The drawing under review shows one solid part. Ordinate dimensions are in mm from its lowest x, y, z. A direction names the side the tool comes from. Round coordinates to 2 decimals unless told otherwise and drop trailing zeros. Write each loop counter-clockwise with the first axis right and the second up, starting at its lowest first coordinate (ties: lowest second). Pieces come first, ordered by that corner, then holes. Notation, with made-up numbers: (66, 57.5) -> (89, 57.5) arc R11 cw to (89, 71.5) -> close; hole circle Ø7 at (-13, 52.25). An arc over 180 degrees is marked (long way). Write item = value, one per line. Start each with the question number.
Item 1: Add section B-B, the plane z = 9.5. State the section outline as (x, y) points, then the cut area to 3 significant figures.
Item 2: Add section C-C, the plane y = 21. State the section outline as (x, z) points.
Item 3: Add section A-A, the plane y = 50. State the section outline as (x, z) points, then the cut area to 3 significant figures.
Item 4: Mouldability with a two-part tool opening along Z and no side actions: class the marked faces 3, 4, 5 and 6 as released by +Z, released by -Z, zero draft, split by the parting line, or undercut.
Item 5: Machinability: for the marked faces 1 and 2, which of the approach directions +Z, -Z, +X, -X, +Y, -Y give a long, thin tool a straight path to every point of the face, cutting with its end or side? Answer none if there is none.
Item 6: To check wall thickness, follow L1, parallel to Z at x = 4.25, y = 21.5; L2, parallel to Z at x = 0.85, y = 50. State the ranges of each line that lie inside material, in increasing order.
Item 7: Add section D-D, the plane x = 9.5. State the section outline as (y, z) points.
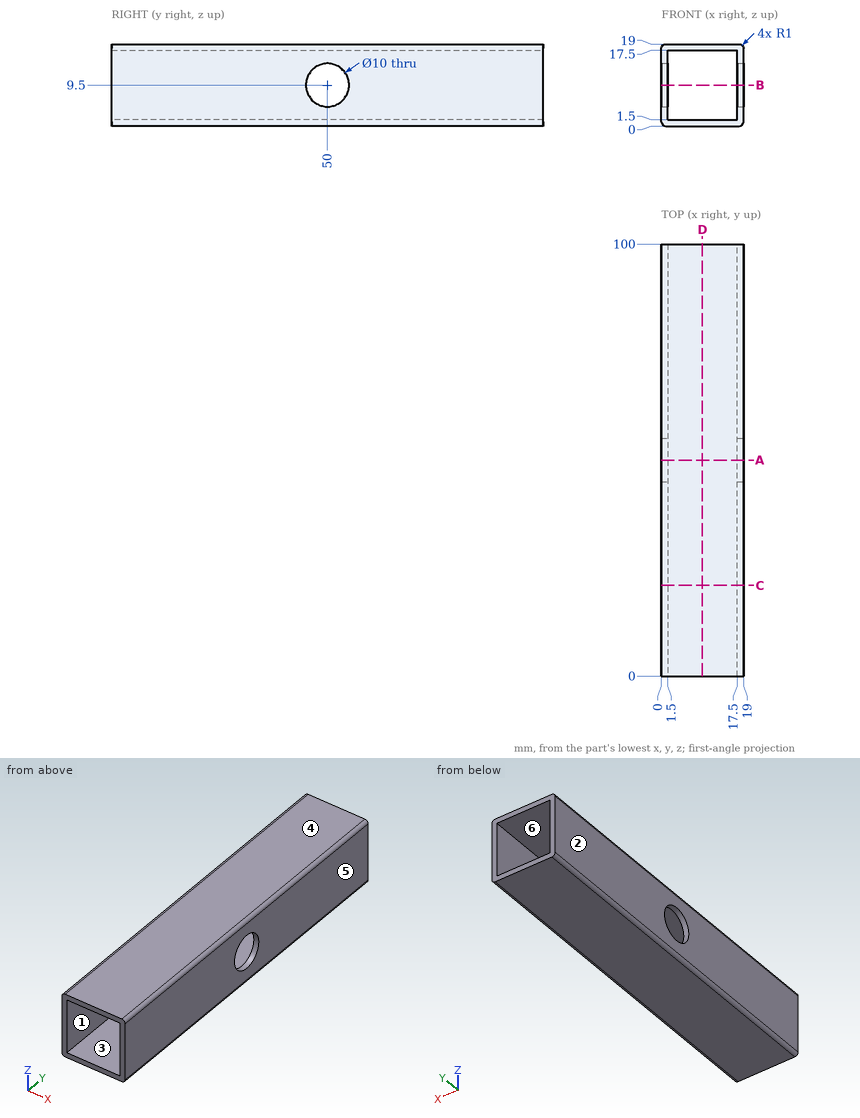
Result set:
q1.outline = (0, 0) -> (1.5, 0) -> (1.5, 45) -> (0, 45) -> close; (0, 55) -> (1.5, 55) -> (1.5, 100) -> (0, 100) -> close; (17.5, 0) -> (19, 0) -> (19, 45) -> (17.5, 45) -> close; (17.5, 55) -> (19, 55) -> (19, 100) -> (17.5, 100) -> close
q1.area = 270 mm²
q2.outline = (0, 1) arc R1 ccw to (1, 0) -> (18, 0) arc R1 ccw to (19, 1) -> (19, 18) arc R1 ccw to (18, 19) -> (1, 19) arc R1 ccw to (0, 18) -> close; hole (1.5, 1.5) -> (17.5, 1.5) -> (17.5, 17.5) -> (1.5, 17.5) -> close
q3.outline = (0, 1) arc R1 ccw to (1, 0) -> (18, 0) arc R1 ccw to (19, 1) -> (19, 4.5) -> (17.5, 4.5) -> (17.5, 1.5) -> (1.5, 1.5) -> (1.5, 4.5) -> (0, 4.5) -> close; (0, 14.5) -> (1.5, 14.5) -> (1.5, 17.5) -> (17.5, 17.5) -> (17.5, 14.5) -> (19, 14.5) -> (19, 18) arc R1 ccw to (18, 19) -> (1, 19) arc R1 ccw to (0, 18) -> close
q3.area = 74.1 mm²
q4.face_3 = undercut
q4.face_4 = released by +Z
q4.face_5 = zero draft
q4.face_6 = undercut
q5.face_1 = +Y, -Y
q5.face_2 = +Z, -Z, -X, +Y, -Y
q6.L1 = 0 to 1.5, 17.5 to 19
q6.L2 = 0.01 to 4.5, 14.5 to 18.99
q7.outline = (0, 0) -> (100, 0) -> (100, 1.5) -> (0, 1.5) -> close; (0, 17.5) -> (100, 17.5) -> (100, 19) -> (0, 19) -> close
